The drawing under review shows one solid part. Ordinate dimensions are in mm from its lowest x, y, z. A direction names the side the tool comes from. Coordinates: 2 decimals unless noted, no trailing zeros. Order: outer loops, then holes, each group sorted by start corner. A loop starts at its lowest first (then second) coordinate and runs counter-clockwise, first axis right, second up. Notation, with made-up numbers: (89.5, -17) -> (128.5, -17) arc R6 ccw to (128.5, -11) -> close; hole circle Ø3 at (65, 2). An arc over 180 degrees is marked (long way). Write item = value, one per line.
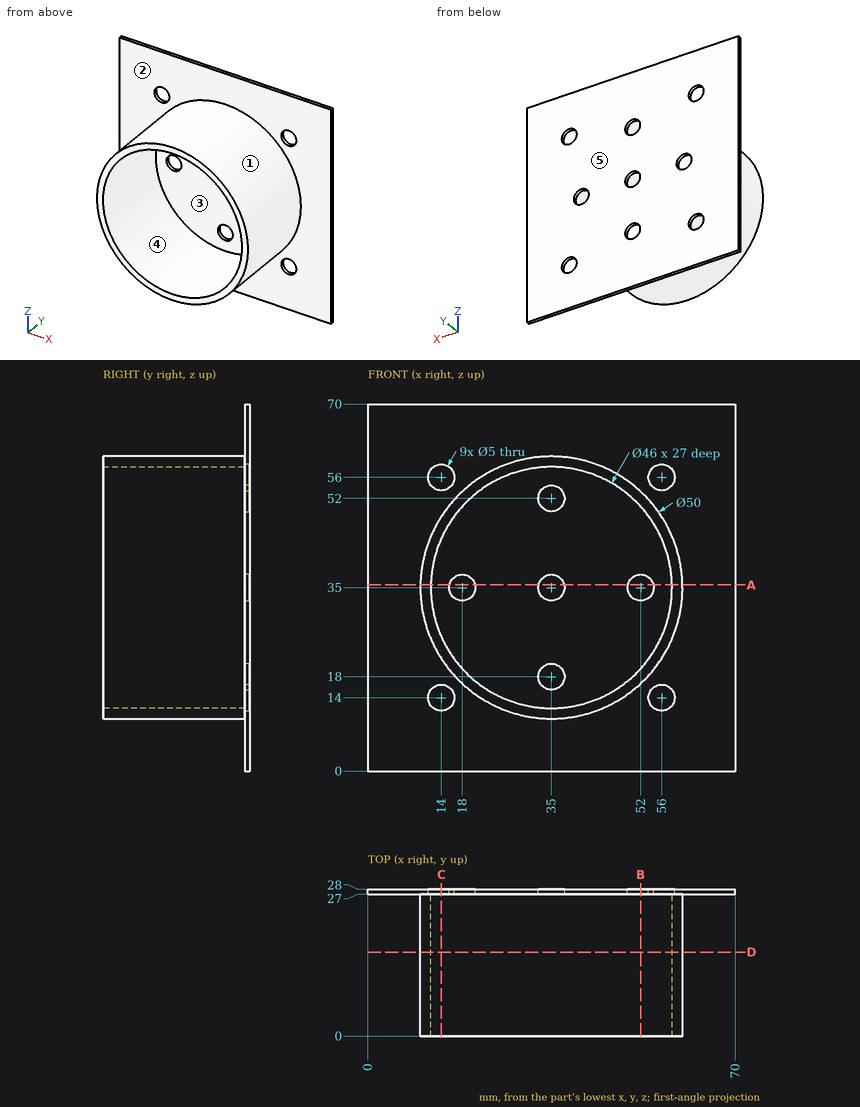
(1) Insertion check: pin 1 (2 mm diameter, centred on x = 16, y = 4, fed in from -Z); pin 2 (6.5 mm diameter, centred on x = 35, z = 35, fed in from -Y); pin 3 (10 mm diameter, centred on x = 57.5, y = 3, fed in from -Z). Each pin has a flat end and moves straight along its axis. Give the tip position at first contact, or say it passes through.
Report:
pin_1 = 17.65
pin_2 = 27
pin_3 = 17.15
(2) We need section D-D (y = 16). Write out the cut boundary in (x, z), and give its area (3 significant figures).
Report:
outline = circle Ø50 at (35, 35); hole circle Ø46 at (35, 35)
area = 302 mm²
(3) For the marked faces 4 and 5, list the 3-axis set-ups (+Z, -Z, +X, -X, +Y, -Y) from which the entire face can be reached by the end or side of a thin tool; tool diameter is ignored.
Report:
face_4 = -Y
face_5 = +Z, -Z, +X, -X, +Y
(4) We need section A-A (z = 35.5). Write out the cut boundary in (x, y) (3 decimals), and give its area (3 significant figures).
Report:
outline = (0, 27) -> (10.005, 27) -> (10.005, 0) -> (12.005, 0) -> (12.005, 27) -> (15.551, 27) -> (15.551, 28) -> (0, 28) -> close; (20.449, 27) -> (32.551, 27) -> (32.551, 28) -> (20.449, 28) -> close; (37.449, 27) -> (49.551, 27) -> (49.551, 28) -> (37.449, 28) -> close; (54.449, 27) -> (57.995, 27) -> (57.995, 0) -> (59.995, 0) -> (59.995, 27) -> (70, 27) -> (70, 28) -> (54.449, 28) -> close
area = 163 mm²
(5) We need section C-C (x = 14). Write out the cut boundary in (y, z).
Report:
outline = (0, 21.44) -> (27, 21.44) -> (27, 16.5) -> (28, 16.5) -> (28, 53.5) -> (27, 53.5) -> (27, 48.56) -> (0, 48.56) -> (0, 44.38) -> (27, 44.38) -> (27, 25.62) -> (0, 25.62) -> close; (27, 0) -> (28, 0) -> (28, 11.5) -> (27, 11.5) -> close; (27, 58.5) -> (28, 58.5) -> (28, 70) -> (27, 70) -> close
(6) The part is to be moulded in two halves that separate along Z. For the marked faces 1, 2 and 3, say which applies: released by +Z, released by -Z, zero draft, split by the parting line, or undercut.
Report:
face_1 = split by the parting line
face_2 = zero draft
face_3 = undercut
(7) For L1, parallel to X at y = 27.2, z = 35; L2, parallel to X at y = 27.35, z = 56; L3, parallel to Y at x = 40.5, z = 59.5, list the stretches that pass through material, from the lowest coordinate up.
Report:
L1 = 0 to 15.5, 20.5 to 32.5, 37.5 to 49.5, 54.5 to 70
L2 = 0 to 11.5, 16.5 to 53.5, 58.5 to 70
L3 = 27 to 28
(8) We need section B-B (x = 52). Write out the cut boundary in (y, z).
Report:
outline = (0, 16.67) -> (27, 16.67) -> (27, 0) -> (28, 0) -> (28, 32.5) -> (27, 32.5) -> (27, 19.51) -> (0, 19.51) -> close; (0, 50.49) -> (27, 50.49) -> (27, 37.5) -> (28, 37.5) -> (28, 70) -> (27, 70) -> (27, 53.33) -> (0, 53.33) -> close
